Build history of the part. All positions in model axes, mm. A direction names the side the tool comes from. Round coordinates to 2 decimals unless told otherwise and drop trailing zeros. Write each loop counter-clockwise with the first axis right and the second up, starting at its lowest first coordinate (ties: lowest second). Pieces come first, ordered by that corner, then holes. Notation, with made-up numbers: M -38.5,-25 L 4.5,-25 A16 ccw 4.5,-11 Z; hole C 30,6 d11. An arc over 180 degrees is marked long. Write item = value, one per line.
Autodesk Inventor part; units mm, degrees
ref_plane "YZ Plane" through (0, 0, 0) normal (1, 0, 0) x (0, 1, 0)
ref_plane "XZ Plane" through (0, 0, 0) normal (0, 1, 0) x (-1, 0, 0)
ref_plane "XY Plane" through (0, 0, 0) normal (0, 0, 1) x (1, 0, 0)
sketch "Sketch1" plane through (0, 0, 0) normal (0, 1, 0) x (-1, 0, 0)
  line L0 (0, 0) -> (40, 0)
  line L1 (40, 0) -> (40, -30)
  line L2 (40, -30) -> (0, -30)
  line L3 (0, 0) -> (0, -30)
  dimension "d0" = 40
  dimension "d1" = 30
extrude "Extrusion1" add sketch "Sketch1" along normal blind 10
sketch "Sketch2" plane through (0, 0, -30) normal (0, 0, -1) x (-1, 0, 0)
  line L0 (0, 0) -> (0, 10)
  line L1 (0, 10) -> (3.5, 10)
  line L2 (0, 10) -> (40, 10)
  line L3 (3.5, 10) -> (0, 6.5)
  line L4 (0, 6.5) -> (0, 10)
  line L5 (0, 10) -> (3.5, 10)
  dimension "d4" = 3.5
  dimension "d5" = 45
extrude "Extrusion2" cut sketch "Sketch2" against normal blind 17.5
sketch "Sketch3" plane through (0, 0, -30) normal (0, 0, -1) x (-1, 0, 0)
  line L0 (40, 0) -> (40, 10)
  line L1 (40, 10) -> (36.5, 10)
  line L2 (40, 10) -> (0, 10)
  line L3 (36.5, 10) -> (40, 6.5)
  line L4 (40, 6.5) -> (40, 10)
  point P0 (0, 0)
  dimension "d8" = 3.5
  dimension "d9" = 45
extrude "Extrusion3" cut sketch "Sketch3" against normal blind 17.5
sketch "Sketch4" plane through (0, 0, -30) normal (0, 0, -1) x (-1, 0, 0)
  line L0 (0, 0) -> (40, 0)
  line L1 (3.5, 10) -> (0, 6.5)
  line L2 (0, 0) -> (0, 6.5)
  line L3 (3.5, 10) -> (36.5, 10)
  line L4 (0, 6.5) -> (3.5, 10)
  line L5 (40, 6.5) -> (36.5, 10)
  line L6 (3.5, 10) -> (36.5, 10)
  line L7 (36.5, 10) -> (40, 6.5)
  line L8 (40, 0) -> (40, 10)
  line L9 (40, 6.5) -> (40, 0)
  line L10 (40, 0) -> (0, 0)
extrude "Extrusion4" add sketch "Sketch4" along normal blind 30
sketch "Sketch5" plane through (0, 0, -60) normal (0, 0, -1) x (-1, 0, 0)
  line L0 (36.5, 10) -> (3.5, 10)
  line L1 (3.5, 10) -> (0, 6.5)
  line L2 (3.5, 10) -> (0, 6.5)
  line L3 (0, 0) -> (0, 10)
  line L4 (0, 6.5) -> (0, 10)
  line L5 (0, 10) -> (3.5, 10)
  line L6 (36.5, 10) -> (40, 10)
  line L7 (36.5, 10) -> (40, 10)
  line L8 (40, 10) -> (40, 6.5)
  line L9 (40, 6.5) -> (36.5, 10)
extrude "Extrusion5" add sketch "Sketch5" against normal blind 12.5 contours L1 L3 L5
sketch "Sketch6" plane through (0, 0, -60) normal (0, 0, -1) x (-1, 0, 0)
  line L0 (40, 6.5) -> (36.5, 10)
  line L1 (40, 10) -> (0, 10)
  line L2 (36.5, 10) -> (40, 10)
  line L3 (40, 10) -> (40, 6.5)
  line L4 (40, 10) -> (40, 6.5)
  line L5 (40, 6.5) -> (36.5, 10)
  point P0 (0, 0)
extrude "Extrusion6" add sketch "Sketch6" against normal blind 12.5
fillet "Fillet1" radius 2.25 2 edges at (-40, 5, 0) (0, 5, 0)
sketch "Sketch7" plane through (0, 10, 0) normal (0, 1, 0) x (1, 0, 0)
  line L0 (-37.75, 0) -> (-2.25, 0)
  circle A0 centre (-20, 30) radius 13
  point P0 (0, 0)
  dimension "d21" = 26
extrude "Extrusion7" cut sketch "Sketch7" against normal blind 10
sketch "Sketch8" plane through (-37.75, 0, 0) normal (0, 0, 1) x (1, 0, 0)
  line L0 (-2.25, 10) -> (-2.25, 0)
  line L1 (-2.25, 10) -> (17.75, 10)
  line L2 (4.75, 10) -> (30.75, 10)
  line L3 (17.75, 10) -> (17.75, 6.8)
  circle A0 centre (17.75, 6.8) radius 1.36
  point P0 (37.75, 0)
  dimension "d24" = 20
  dimension "d25" = 3.2
  dimension "d26" = 2.72
extrude "Extrusion8" cut sketch "Sketch8" against normal blind 11
sketch "Sketch9" plane through (-20, 6.8, -11) normal (0, 0, 1) x (1, 0, 0)
  circle A0 centre (0, 0) radius 1.785
  point P0 (20, -6.8)
  dimension "d29" = 3.57
extrude "Extrusion9" cut sketch "Sketch9" against normal blind 10
sketch "Sketch10" plane through (0, 10, 0) normal (0, 1, 0) x (1, 0, 0)
  point P0 (0, 0)
sketch "Sketch11" plane through (0, 10, 0) normal (0, 1, 0) x (1, 0, 0)
  point P0 (0, 0)
sketch "Sketch12" plane through (0, 0, 0) normal (0, -1, 0) x (1, 0, 0)
  line L0 (-18.215, -11) -> (-18.215, -17.1231)
  line L1 (-18.215, -17.1231) -> (-21.785, -17.1231)
  line L2 (-21.785, -11) -> (-21.785, -17.1231)
  line L3 (-18.215, -11) -> (-21.785, -11)
  line L4 (-21.785, -11) -> (-18.215, -11)
  line L5 (-18.215, -11) -> (-18.215, -17.1231)
  point P0 (0, 0)
extrude "Extrusion10" cut sketch "Sketch12" against normal blind 6.8
sketch "Sketch13" plane through (0, 0, 0) normal (0, -1, 0) x (1, 0, 0)
  line L0 (-21.36, 0) -> (-21.36, -11)
  line L1 (-21.36, -11) -> (-21.36, 0)
  line L2 (-37.75, 0) -> (-2.25, 0)
  line L3 (-21.36, 0) -> (-18.64, 0)
  line L4 (-21.36, 0) -> (-18.64, 0)
  line L5 (-18.64, 0) -> (-18.64, -11)
  line L6 (-18.64, -11) -> (-18.64, 0)
  line L7 (-18.64, -11) -> (-21.36, -11)
  point P0 (0, 0)
extrude "Extrusion11" cut sketch "Sketch13" against normal blind 6.8
properties part number "NewSWTop"
1. Band-saw the part on D-D (x = -29.5). List the corners of the cut face in (y, z).
Responses:
outline = M 0,-60 L 10,-60 L 10,-38.87 L 0,-38.87 Z; M 0,-21.13 L 10,-21.13 L 10,0 L 0,0 Z
2. Band-saw the part on B-B (z = -30). List the corners of the cut face in (x, y), plus the area to 3 significant figures.
Responses:
outline = M -40,0 L -33,0 L -33,10 L -36.5,10 L -40,6.5 Z; M -7,0 L 0,0 L 0,6.5 L -3.5,10 L -7,10 Z
area = 128 mm²
3. Mould opens along Z. For faces 1 (the face through (-0.68, 5.07, -0.64)), 2 (the face through (-1, 9, -12.5)), 3 (the face through (-21.36, 3, -5)) say: pulls with the +Z half, pulls with the -Z half, needs draft (parallel to the pull), parting line crosses it, or undercut.
Responses:
face_1 = pulls with the +Z half
face_2 = undercut
face_3 = needs draft
4. Tool access for faces 4 (the face through (-1.8, 8.3, -29.8)), 5 (the face through (-18.4, 4.9, -11)), 6 (the face through (-38.3, 8.2, -29.8)), 7 (the face through (-18.64, 3, -5)): list every direction of +Z, -Z, +X, -X, +Y, -Y with a clear straight run to the whole face (end or side of a thin tool).
Responses:
face_4 = +X, +Y
face_5 = -Y
face_6 = -X, +Y
face_7 = +Z, -Y
5. Band-saw the part on A-A (x = -20). List the corners of the cut face in (y, z) (3 decimals), plus the area to 3 significant figures.
Responses:
outline = M 0,-60 L 10,-60 L 10,-43 L 0,-43 Z; M 8.16,-11 L 8.585,-11 L 8.585,-17 L 10,-17 L 10,0 L 8.16,0 Z
area = 199 mm²
6. Flat gauge pin, fed straight in: pin 1 (6 mm diameter, centred on y = 6, z = -36, fed in from +X). Where does the tip first touch, or does it go through?
Responses:
pin_1 = 0
7. Band-saw the part on C-C (z = -15.5). List the corners of the cut face in (x, y) (3 decimals).
Responses:
outline = M -40,0 L -21.785,0 L -21.785,6.8 A1.785 cw -18.215,6.8 L -18.215,0 L 0,0 L 0,6.5 L -3.5,10 L -36.5,10 L -40,6.5 Z
8. Probe probe 1 along X at (y, z) = (2.5, -30); probe 2 along X at (y, z) = (2.75, -16.5) (3 decimals); probe 3 along Z at (x, y) = (-20, 7.5). List the from-to ranges inside material, lowest first.
Responses:
probe_1 = -40 to -33, -7 to 0
probe_2 = -40 to -21.785, -18.215 to 0
probe_3 = -60 to -43
